Geometry: see drawing. Coordinates: mm, zero at the bounding-box minimum. Give positions to 0.01 mm unless a question says otherwise; leave off trailing zeros. Write each loop counter-clockwise with the first axis right and the second up, starting at its lowest first coordinate (ties: lowest second). Pieces come first, ordered by that corner, then holes. Notation, with made-up numbers: (-3, -16.75) - (50, -16.75) arc R25 ccw to (50, 2.25) - close; hole circle Ø3 at (-11, 17.25). An arc over 180 degrees is marked (long way). Use a Markdown table: item, result. Add a question column.
1. Section query C-C, the plane z = 20. Return loops of the section in (x, y), plus the area to 3 significant figures.
2. Material intervals for probe 1 along Z at (x, y) = (42.5, 2.3); probe 2 along X at (y, z) = (2.05, 94); probe 3 along Z at (x, y) = (40.5, 2.65), sorted ascending.
3. Section query D-D, the plane y = 2.2. Return loops of the section in (x, z), plus the area to 3 significant figures.
4. Section query B-B, the plane x = 70. Return loops of the section in (y, z).
5. Pin query (flat end, axial travel): pin 1 (1.5 mm diameter, centred on y = 1, z = 69, fed in from -X); pin 2 (5.5 mm diameter, centred on x = 42.5, z = 20, fed in from -Y); pin 3 (1.5 mm diameter, centred on x = 7.5, y = 2, fed in from -Z); pin 4 (1 mm diameter, centred on x = 60, y = 1.5, fed in from -Z). Return the tip coordinate at first contact, or that it passes through.
6. Section query A-A, the plane x = 42.5. Return loops of the section in (y, z).
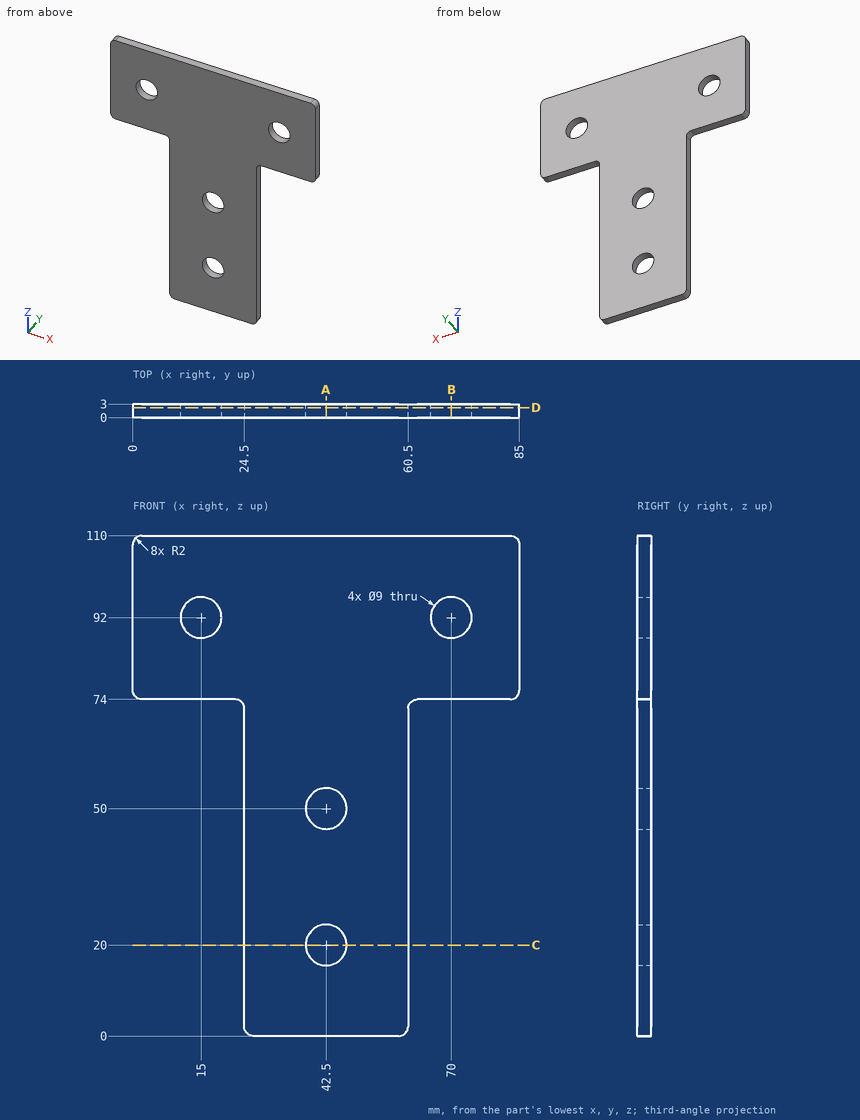
Result sheet:
| question | item | result |
|---|---|---|
| 1 | outline | (24.5, 0) - (38, 0) - (38, 3) - (24.5, 3) - close; (47, 0) - (60.5, 0) - (60.5, 3) - (47, 3) - close |
| 1 | area | 81.0 mm² |
| 2 | probe 1 | z = 0 to 15.5, 24.5 to 45.5, 54.5 to 110 |
| 2 | probe 2 | x = 0 to 10.97, 19.03 to 65.97, 74.03 to 85 |
| 2 | probe 3 | z = 0 to 15.97, 24.03 to 45.97, 54.03 to 110 |
| 3 | outline | (0, 76) arc R2 ccw to (2, 74) - (22.5, 74) arc R2 cw to (24.5, 72) - (24.5, 2) arc R2 ccw to (26.5, 0) - (58.5, 0) arc R2 ccw to (60.5, 2) - (60.5, 72) arc R2 cw to (62.5, 74) - (83, 74) arc R2 ccw to (85, 76) - (85, 108) arc R2 ccw to (83, 110) - (2, 110) arc R2 ccw to (0, 108) - close; hole circle Ø9 at (15, 92); hole circle Ø9 at (42.5, 20); hole circle Ø9 at (42.5, 50); hole circle Ø9 at (70, 92) |
| 3 | area | 5,470 mm² |
| 4 | outline | (0, 74) - (3, 74) - (3, 87.5) - (0, 87.5) - close; (0, 96.5) - (3, 96.5) - (3, 110) - (0, 110) - close |
| 5 | pin 1 | stops at x = 24.5 |
| 5 | pin 2 | passes through |
| 5 | pin 3 | stops at z = 74 |
| 5 | pin 4 | stops at z = 0.27 |
| 6 | outline | (0, 0) - (3, 0) - (3, 15.5) - (0, 15.5) - close; (0, 24.5) - (3, 24.5) - (3, 45.5) - (0, 45.5) - close; (0, 54.5) - (3, 54.5) - (3, 110) - (0, 110) - close |
